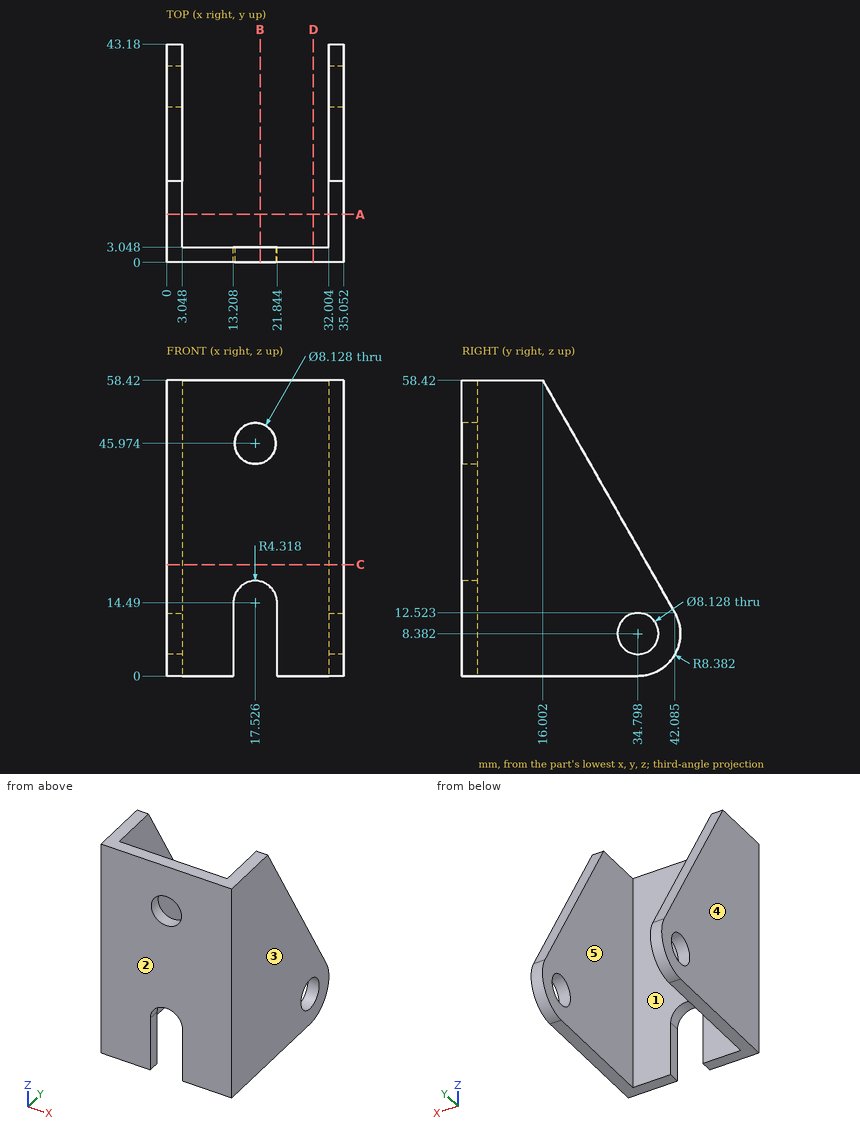
Design review of the part shown in the three views and the two pictorial views. Dimensions are in mm from the part's minimum x, y and z. A direction names the side the tool comes from. Round coordinates to 2 decimals unless told otherwise and drop trailing zeros. Loops run counter-clockwise (first coordinate to the right, second up) from the corner with the lowest first, then second, coordinate; pieces in that order, holes last.
(1) Tool access review of the marked faces 4 and 5: name each direction out of +Z, -Z, +X, -X, +Y, -Y from which nothing blocks a thin tool from reaching the whole face with its end or side.
Returned:
face 4: +Z, -Z, -X, +Y, -Y
face 5: +Z, -Z, +Y
(2) We need section C-C (z = 22). Give the boundary of the cut face in (x, y), plus the area to 3 significant figures.
Returned:
outline: (0, 0) - (35.05, 0) - (35.05, 36.7) - (32, 36.7) - (32, 3.05) - (3.05, 3.05) - (3.05, 36.7) - (0, 36.7) - close
area: 312 mm2
(3) We need section D-D (x = 29). Give the boundary of the cut face in (y, z).
Returned:
outline: (0, 0) - (3.05, 0) - (3.05, 58.42) - (0, 58.42) - close
(4) Mouldability with a two-part tool opening along X and no side actions: class the marked faces 1, 2 and 3 as released by +X, released by -X, zero draft, split by the parting line, or undercut.
Returned:
face 1: undercut
face 2: zero draft
face 3: released by +X
(5) Wall thickness on line 1 along X through (y, z) = (25.5, 9.5); line 2 along Y through (x, z) = (10.5, 13.5): over which ranges is each line inside the solid? List them lowest first.
Returned:
line 1: x = 0 to 3.05, 32 to 35.05
line 2: y = 0 to 3.05
(6) Clearance check with flat-ended pins moving along their axes: P1, Ø3, axis at y = 6, z = 30.5, coming from the -X side; P2, Ø14.5, axis at x = 14.5, z = 39, coming from the +Y side; P3, Ø6, axis at x = 30, z = 22.5, coming from the +Y side (1 decimal); P4, Ø8, axis at x = 7.5, y = 10.5, coming from the +Z side. State where each tip first meets the part, or that it passes through.
Returned:
P1: stops at x = 0
P2: stops at y = 3.05
P3: stops at y = 37.7
P4: passes through
(7) We need section A-A (y = 9.5). Give the boundary of the cut face in (x, z), plus the area to 3 significant figures.
Returned:
outline: (0, 0) - (3.05, 0) - (3.05, 58.42) - (0, 58.42) - close; (32, 0) - (35.05, 0) - (35.05, 58.42) - (32, 58.42) - close
area: 356 mm2
(8) We need section B-B (x = 18.5). Give the boundary of the cut face in (y, z).
Returned:
outline: (0, 18.7) - (3.05, 18.7) - (3.05, 42.03) - (0, 42.03) - close; (0, 49.92) - (3.05, 49.92) - (3.05, 58.42) - (0, 58.42) - close
